Part model, mm, in its own coordinate system. A direction names the side the tool comes from. Coordinates: 2 decimals unless noted, no trailing zeros. Loops run counter-clockwise (first coordinate to the right, second up) from the corner with the lowest first, then second, coordinate; pieces in that order, holes last. Notation, with made-up numbers: (67, 65) - (85, 65) arc R7 ccw to (85, 76) - close; hole circle Ø5 at (10.25, -35.5). An arc over 180 degrees is marked (long way). One line per question, with ' | ' between items. Start each with the question number.
from build123d import *

# Parameters (mm, degrees)
SKETCH1_W           = 100
SKETCH1_H           = 100
BOSS_EXTRUDE1_DEPTH = 170.2
SKETCH2_R           = 38.629656057
CUT_EXTRUDE1_DEPTH  = 39.2
SKETCH3_R           = 26.36678746
BOSS_EXTRUDE2_DEPTH = 39.2


with BuildPart() as part:
    # Sketch1 → Boss-Extrude1 (new body)
    with BuildSketch(Plane(origin=(0, 0, 0), x_dir=(1, 0, 0), z_dir=(0, 1, 0))):
        Rectangle(SKETCH1_W, SKETCH1_H)
    extrude(amount=BOSS_EXTRUDE1_DEPTH)

    # Sketch2 → Cut-Extrude1 (cut)
    with BuildSketch(Plane.XZ):
        with Locations(Location((0, 0, 0), (0, 0, 270))):
            Circle(SKETCH2_R)
    extrude(amount=-CUT_EXTRUDE1_DEPTH, mode=Mode.SUBTRACT)

    # Sketch3 → Boss-Extrude2 (add)
    with BuildSketch(Plane.XZ.offset(-39.2)):
        with Locations(Location((0, 0, 0), (0, 0, 270))):
            Circle(SKETCH3_R)
    extrude(amount=BOSS_EXTRUDE2_DEPTH)


solid = part.part
1) Wall check: line 1 along X through (y, z) = (11, 0); line 2 along Z through (x, y) = (-24.5, 18); line 3 along Z through (x, y) = (7, 25). Give the ranges that are in metal, low to high. Write a range as [from, to].
2) Band-saw the part on D-D on z = 35.5. List the corners of the cut face in (x, y).
3) Tool access for faces 1 (the flat face through (-1, 170.2, -1)), 2 (the cylindrical face through (-16.044, 19.874, 20.924)): list every direction of +Z, -Z, +X, -X, +Y, -Y with a clear straight run to the whole face (end or side of a thin tool).
4) Band-saw the part on C-C on x = 0. List the corners of the cut face in (y, z).
5) Mould opens along Z. For faces 3 (the flat face through (-1, 84, -50)), 4 (the cylindrical face through (11.603, 19.326, -36.846)), 5 (the flat face through (50, 84, 1)), 6 (the flat face through (-25, 39.2, 9)) say: +Z half, -Z half, draft (parallel to the pull), parting line (faces both ways), or undercut.
6) Band-saw the part on A-A on y = 27. List the corners of the cut face in (x, z).
7) Pin check, flat tip, straight feed: pin 1 Ø1.5 at (x, z) = (24.5, -13) entering from -Y. Stop position of the tip, or through.
8) Band-saw the part on B-B on z = 0. List the corners of the cut face in (x, y).
Values found:
1) line 1: [-50, -38.63], [-26.37, 26.37], [38.63, 50] | line 2: [-50, -29.87], [-9.74, 9.74], [29.87, 50] | line 3: [-50, -37.99], [-25.42, 25.42], [37.99, 50]
2) outline: (-50, 0) - (-15.23, 0) - (-15.23, 39.2) - (15.23, 39.2) - (15.23, 0) - (50, 0) - (50, 170.2) - (-50, 170.2) - close
3) face 1: +Z, -Z, +X, -X, +Y | face 2: -Y
4) outline: (0, -50) - (170.2, -50) - (170.2, 50) - (0, 50) - (0, 38.63) - (39.2, 38.63) - (39.2, 26.37) - (0, 26.37) - (0, -26.37) - (39.2, -26.37) - (39.2, -38.63) - (0, -38.63) - close
5) face 3: -Z half | face 4: undercut | face 5: draft | face 6: undercut
6) outline: (-50, -50) - (50, -50) - (50, 50) - (-50, 50) - close; circle Ø52.73 at (0, 0); hole circle Ø77.26 at (0, 0)
7) pin 1: y = 39.2
8) outline: (-50, 0) - (-38.63, 0) - (-38.63, 39.2) - (-26.37, 39.2) - (-26.37, 0) - (26.37, 0) - (26.37, 39.2) - (38.63, 39.2) - (38.63, 0) - (50, 0) - (50, 170.2) - (-50, 170.2) - close
